Could you check a few things on this model? Use its own coordinates, in mm. Coordinates: 2 decimals unless noted, no trailing zeros. Loops run counter-clockwise (first coordinate to the right, second up) from the corner with the lowest first, then second, coordinate; pieces in that order, holes last.
1) Will these pins go through, and if not, where does the flat tip stop? P1, Ø3, axis at x = -43, y = 0, coming from the +Z side; P2, Ø1.5, axis at y = -31.5, z = 2, coming from the -X side.
2) Imagine slicing it at D-D on x = -31. Please give me the cut outline in (y, z).
3) Imagine slicing it at C-C on y = 0. Please give me the cut outline in (x, z), plus the area to 3 significant figures.
4) Imagine slicing it at B-B on z = 0.5. Please give me the cut outline in (x, y), plus the area to 3 significant figures.
5) If I drill on line 1 along Y through (x, z) = (-37, 1.9); line 2 along X through (y, z) = (1, 1.4); line 3 along Y through (x, z) = (-38, 0.3), over which ranges is the centre line in solid material (lowest first)?
6) Imagine slicing it at A-A on x = 0. Please give me the cut outline in (y, z), plus the area to 3 significant figures.
```python
from build123d import *

# Parameters (mm, degrees)
IZIM1_R                     = 1.75
Y_KSEKLIK_EKSTR_ZYON1_DEPTH = 3
Y_KSEKLIK_EKSTR_ZYON2_DEPTH = 3
IZIM4_R                     = 1.75
Y_KSEKLIK_EKSTR_ZYON3_DEPTH = 3
RADYUS1_R                   = 20
IZIM4_3_R                   = 1.75
KES_EKSTR_ZYON1_DEPTH       = 10


with BuildPart() as part:
    # Çizim1 → Yükseklik-Ekstrüzyon1 (new body)
    with BuildSketch(Plane.XY):
        with BuildLine():
            Line((-43, 7.5), (57, 7.5))
            ThreePointArc((57, 7.5), (64.5, 0), (57, -7.5))
            Line((57, -7.5), (-43, -7.5))
            ThreePointArc((-43, -7.5), (-50.5, 0), (-43, 7.5))
        make_face()
        Circle(IZIM1_R, mode=Mode.SUBTRACT)
        with Locations((-43, 0)):
            Circle(IZIM1_R, mode=Mode.SUBTRACT)
        with Locations((57, 0)):
            Circle(IZIM1_R, mode=Mode.SUBTRACT)
    extrude(amount=Y_KSEKLIK_EKSTR_ZYON1_DEPTH)

    # Çizim2 → Yükseklik-Ekstrüzyon2 (add)
    with BuildSketch(Plane(origin=(0, 0, 0), x_dir=(-1, 0, 0), z_dir=(0, 0, -1))):
        with BuildLine():
            ThreePointArc((-57, -7.5), (-64.5, 0), (-57, 7.5))
            Line((-57, 7.5), (-61.290238096, 7.5))
            ThreePointArc((-61.290238096, 7.5), (-90.835057362, -12.499091059), (-87.794753659, -48.04647552))
            ThreePointArc((-87.794753659, -48.04647552), (-66.485762327, -18.707163802), (-32, -7.5))
            Line((-32, -7.5), (-57, -7.5))
        make_face()
    extrude(amount=-Y_KSEKLIK_EKSTR_ZYON2_DEPTH)

    # Çizim4 → Yükseklik-Ekstrüzyon3 (add)
    with BuildSketch(Plane.XY):
        with BuildLine():
            Line((-33.824470976, -15.071432033), (-22.668001232, -7.5))
            Line((-22.668001232, -7.5), (-22.668001232, 7.5))
            Line((-22.668001232, 7.5), (-43, 7.5))
            ThreePointArc((-43, 7.5), (-49.765006227, 3.23800722), (-48.841370401, -4.704082465))
            Line((-48.841370401, -4.704082465), (-41.404337559, -13.93913815))
            ThreePointArc((-41.404337559, -13.93913815), (-37.835472898, -15.985175384), (-33.824470976, -15.071432033))
        make_face()
        with Locations((-37, -10.392304845)):
            Circle(IZIM4_R, mode=Mode.SUBTRACT)
        with Locations((-43, 0)):
            Circle(IZIM4_R, mode=Mode.SUBTRACT)
        with Locations((-31, 0)):
            Circle(IZIM4_R, mode=Mode.SUBTRACT)
    extrude(amount=Y_KSEKLIK_EKSTR_ZYON3_DEPTH)

    # Radyus1
    radyus1_edges = [part.edges().sort_by_distance(p)[0] for p in [
        (-22.668001232, -7.5, 1.5),
    ]]
    fillet(radyus1_edges, radius=RADYUS1_R)

    # Çizim4<3> → Kes-Ekstrüzyon1 (cut)
    with BuildSketch(Plane.XY):
        with Locations((-31, 0)):
            Circle(IZIM4_3_R)
    extrude(amount=KES_EKSTR_ZYON1_DEPTH, mode=Mode.SUBTRACT)

    # Pah2
    # the kernel refuses this chamfer: 3, 2.517298894 mm, written as the material it takes off along each edge
    with BuildSketch(Plane(origin=(32, -66.161957074, 0), x_dir=(0.9999969206836817, -0.0024816573402179206, 0), z_dir=(-0.0024816573402179206, -0.9999969206836817, 0))) as pah2_piece_1:
        with BuildLine():
            Line((61.753882408, -0.077134513), (58.570031741, 2.594433407))
            Line((58.570031741, 2.594433407), (58.510031741, 2.594433407))
            ThreePointArc((58.510031741, 2.594433407), (58.601957074, 1.297216703), (58.601957074, 0))
            Line((58.601957074, 0), (58.661957074, -0.06))
            ThreePointArc((58.661957074, -0.06), (60.207919741, -0.06), (61.753882408, -0.137134513))
            Line((61.753882408, -0.137134513), (61.753882408, -0.077134513))
        make_face()
    revolve(axis=Axis((32, -66.161957074, 0), (0, 0, 1)), revolution_arc=90.142188638, mode=Mode.SUBTRACT)
    with BuildSketch(Plane(origin=(-43, 7.5, 0), x_dir=(0, -0.9996889667359941, -0.024939322090234348), z_dir=(1, 0, 0))) as pah2_piece_2:
        with BuildLine():
            Line((3.092887324, 0), (-0.156600152, -2.591333896))
            Line((-0.156600152, -2.591333896), (-0.21658149, -2.589837537))
            ThreePointArc((-0.21658149, -2.589837537), (-0.092333043, -1.295316866), (-0.059981338, 0.001496359))
            Line((-0.059981338, 0.001496359), (0.001496359, 0.059981338))
            ThreePointArc((0.001496359, 0.059981338), (1.54697818, 0.021426077), (3.094383683, 0.059981338))
            Line((3.094383683, 0.059981338), (3.092887324, 0))
        make_face()
    extrude(amount=122.84756204, mode=Mode.SUBTRACT)
    with BuildSketch(Plane(origin=(-48.841370401, -4.704082465, 0), x_dir=(0.7786071387098311, 0.6270159118904154, -0.024939322090234337), z_dir=(0.6272109953735269, -0.7788493867767694, 0))) as pah2_piece_3:
        with BuildLine():
            Line((3.092887324, 0), (-0.156600152, 2.591333896))
            Line((-0.156600152, 2.591333896), (-0.21658149, 2.589837537))
            ThreePointArc((-0.21658149, 2.589837537), (-0.092333043, 1.295316866), (-0.059981338, -0.001496359))
            Line((-0.059981338, -0.001496359), (0.001496359, -0.059981338))
            ThreePointArc((0.001496359, -0.059981338), (1.54697818, -0.021426077), (3.094383683, -0.059981338))
            Line((3.094383683, -0.059981338), (3.092887324, 0))
        make_face()
    extrude(amount=11.857306228, mode=Mode.SUBTRACT)
    with BuildSketch(Plane(origin=(-37, -10.392304845, 0), x_dir=(-0.7788493867767683, -0.6272109953735282, 0), z_dir=(-0.6272109953735282, 0.7788493867767683, 0))) as pah2_piece_4:
        with BuildLine():
            Line((2.563003121, -0.077134513), (5.746853788, 2.594433407))
            Line((5.746853788, 2.594433407), (5.806853788, 2.594433407))
            ThreePointArc((5.806853788, 2.594433407), (5.714928454, 1.297216703), (5.714928454, 0))
            Line((5.714928454, 0), (5.654928454, -0.06))
            ThreePointArc((5.654928454, -0.06), (4.108965788, -0.06), (2.563003121, -0.137134513))
            Line((2.563003121, -0.137134513), (2.563003121, -0.077134513))
        make_face()
    revolve(axis=Axis((-37, -10.392304845, 0), (0, 0, 1)), revolution_arc=85.318453593, mode=Mode.SUBTRACT)
    with BuildSketch(Plane(origin=(-33.824470976, -15.071432033, 0), x_dir=(-0.5613760376690521, 0.8271849699702446, -0.024939322090234337), z_dir=(0.8274423320595619, 0.5615506986157474, 0))) as pah2_piece_5:
        with BuildLine():
            Line((3.092887324, 0), (-0.156600152, 2.591333896))
            Line((-0.156600152, 2.591333896), (-0.21658149, 2.589837537))
            ThreePointArc((-0.21658149, 2.589837537), (-0.092333043, 1.295316866), (-0.059981338, -0.001496359))
            Line((-0.059981338, -0.001496359), (0.001496359, -0.059981338))
            ThreePointArc((0.001496359, -0.059981338), (1.54697818, -0.021426077), (3.094383683, -0.059981338))
            Line((3.094383683, -0.059981338), (3.092887324, 0))
        make_face()
    extrude(amount=7.337322676, mode=Mode.SUBTRACT)
    with BuildSketch(Plane(origin=(-43, 0, 0), x_dir=(-0.7788493867767701, -0.6272109953735259, 0), z_dir=(0.6272109953735259, -0.7788493867767701, 0))) as pah2_piece_6:
        with BuildLine():
            Line((4.408074667, 0.077134513), (7.591925333, -2.594433407))
            Line((7.591925333, -2.594433407), (7.651925333, -2.594433407))
            ThreePointArc((7.651925333, -2.594433407), (7.56, -1.297216703), (7.56, 0))
            Line((7.56, 0), (7.5, 0.06))
            ThreePointArc((7.5, 0.06), (5.954037333, 0.06), (4.408074667, 0.137134513))
            Line((4.408074667, 0.137134513), (4.408074667, 0.077134513))
        make_face()
    revolve(axis=Axis((-43, 0, 0), (0, 0, -1)), revolution_arc=128.844653269, mode=Mode.SUBTRACT)
    with BuildSketch(Plane(origin=(32, -7.5, 0), x_dir=(0, -0.035409536913662706, 0.9993728857116145), z_dir=(-1, 0, 0))) as pah2_piece_7:
        with BuildLine():
            Line((2.596061434, 0), (-0.186569785, 3.087255045))
            Line((-0.186569785, 3.087255045), (-0.246532158, 3.085130473))
            ThreePointArc((-0.246532158, 3.085130473), (-0.114704195, 1.542868599), (-0.059962373, -0.002124572))
            Line((-0.059962373, -0.002124572), (0.002124572, -0.059962373))
            ThreePointArc((0.002124572, -0.059962373), (1.298527772, -0.01402853), (2.598186006, -0.059962373))
            Line((2.598186006, -0.059962373), (2.596061434, 0))
        make_face()
    extrude(amount=48.522245618, mode=Mode.SUBTRACT)
    with BuildSketch(Plane(origin=(-16.522245618, -27.5, 0), x_dir=(0, 1, 0), z_dir=(1, 0, 0))) as pah2_piece_8:
        with BuildLine():
            Line((23.091925333, -0.077134513), (19.908074667, 2.594433407))
            Line((19.908074667, 2.594433407), (19.848074667, 2.594433407))
            ThreePointArc((19.848074667, 2.594433407), (19.94, 1.297216703), (19.94, 0))
            Line((19.94, 0), (20, -0.06))
            ThreePointArc((20, -0.06), (21.545962667, -0.06), (23.091925333, -0.137134513))
            Line((23.091925333, -0.137134513), (23.091925333, -0.077134513))
        make_face()
    revolve(axis=Axis((-16.522245618, -27.5, 0), (0, 0, 1)), revolution_arc=34.163106862, mode=Mode.SUBTRACT)


solid = part.part
```
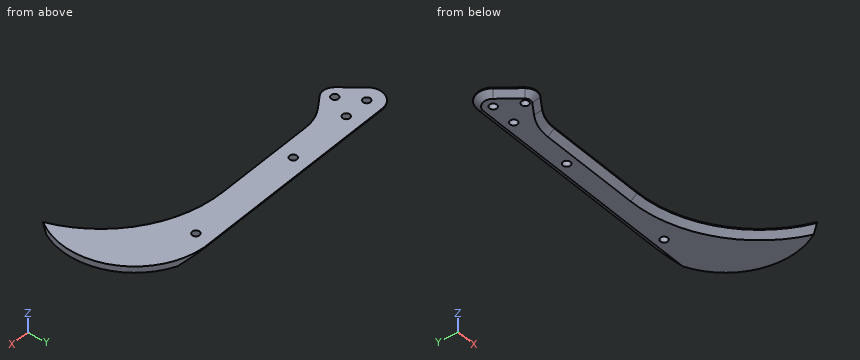
Filled in:
1. P1: passes through
1. P2: stops at x = 78.92
2. outline: (-13.15, 2.52) - (-9.53, 0) - (-1.75, 0) - (-1.75, 3) - (-13.15, 3) - close; (1.75, 0) - (4.5, 0) - (7.5, 2.52) - (7.5, 3) - (1.75, 3) - close
3. outline: (-50.5, 2.52) - (-47.5, 0) - (-44.75, 0) - (-44.75, 3) - (-50.5, 3) - close; (-41.25, 0) - (-32.75, 0) - (-32.75, 3) - (-41.25, 3) - close; (-29.25, 0) - (-1.75, 0) - (-1.75, 3) - (-29.25, 3) - close; (1.75, 0) - (55.25, 0) - (55.25, 3) - (1.75, 3) - close; (58.75, 0) - (80.85, 0) - (80.85, 3) - (58.75, 3) - close
3. area: 348 mm2
4. outline: (-46.97, -3.2) - (-39.53, -12.43) arc R3.25 ccw to (-35.17, -13.08) - (-29.1, -8.96) arc R22.4 cw to (-16.52, -5.1) - (32, -5.1) arc R61.07 cw to (89.45, -45.47) arc R35.25 ccw to (72, 5.1) - (-43, 5.1) arc R5.1 ccw to start; hole circle Ø3.5 at (-43, 0); hole circle Ø3.5 at (-37, -10.39); hole circle Ø3.5 at (-31, 0); hole circle Ø3.5 at (0, 0); hole circle Ø3.5 at (57, 0)
4. area: 2,100 mm2
5. line 1: y = -15.31 to -12.14, -8.64 to 6.76
5. line 2: x = -49.09 to -44.44, -41.56 to -32.44, -29.56 to -1.44, 1.44 to 55.56, 58.44 to 79.52
5. line 3: y = -13.23 to -11.83, -8.96 to 4.86
6. outline: (-7.5, 2.52) - (-4.5, 0) - (-1.75, 0) - (-1.75, 3) - (-7.5, 3) - close; (1.75, 0) - (4.5, 0) - (7.5, 2.52) - (7.5, 3) - (1.75, 3) - close
6. area: 26.9 mm2
